from build123d import *

# Parameters (mm, degrees)
BODY_DEPTH                    = 6.35
HANDLE_DEPTH                  = 6.35
SKETCH11_R                    = 5
LOCKING_MECHANISM_HOLES_DEPTH = 6.36
FILLET1_R                     = 40
FILLET2_R                     = 40
SKETCH12_W                    = 10
SKETCH12_H                    = 30
BOSS_EXTRUDE1_DEPTH           = 4


with BuildPart() as part:
    # Sketch1 → Body (new body)
    with BuildSketch(Plane(origin=(0, 0, 0), x_dir=(1, 0, 0), z_dir=(0, 1, 0))):
        Polygon((0, 0), (294, 0), (336.996020767, 43.003978862), (336.996020767, 337.003978862), (217, 456.999999629), (77, 456.999999629), (-42.996020767, 337.003978862), (-42.996020767, 43.003978862), align=None)
    extrude(amount=BODY_DEPTH)

    # Sketch2 → Handle (cut)
    with BuildSketch(Plane(origin=(0, 6.35, 0), x_dir=(1, 0, 0), z_dir=(0, 1, 0))):
        with BuildLine():
            Line((112.35, 441.799999629), (181.65, 441.799999629))
            ThreePointArc((181.65, 441.799999629), (197.5, 425.949999629), (181.65, 410.099999629))
            Line((181.65, 410.099999629), (112.35, 410.099999629))
            ThreePointArc((112.35, 410.099999629), (96.5, 425.949999629), (112.35, 441.799999629))
        make_face()
    extrude(amount=-HANDLE_DEPTH, mode=Mode.SUBTRACT)

    # Sketch11 → Locking Mechanism Holes (cut)
    with BuildSketch(Plane(origin=(0, 6.35, 0), x_dir=(1, 0, 0), z_dir=(0, 1, 0))):
        with Locations(Location((221.65, 421.999999629, 0), (0, 0, 270))):
            Circle(SKETCH11_R)
        with Locations(Location((72.35, 421.999999629, 0), (0, 0, 270))):
            Circle(SKETCH11_R)
    extrude(amount=-LOCKING_MECHANISM_HOLES_DEPTH, mode=Mode.SUBTRACT)

    # Fillet1
    fillet1_edges = [part.edges().sort_by_distance(p)[0] for p in [
        (77, 3.175, -456.999999629),
        (217, 3.175, -456.999999629),
    ]]
    fillet(fillet1_edges, radius=FILLET1_R)

    # Fillet2
    fillet2_edges = [part.edges().sort_by_distance(p)[0] for p in [
        (-42.996020767, 3.175, -43.003978862),
        (-42.996020767, 3.175, -337.003978862),
        (336.996020767, 3.175, -337.003978862),
        (336.996020767, 3.175, -43.003978862),
        (294, 3.175, 0),
        (0, 3.175, 0),
    ]]
    fillet(fillet2_edges, radius=FILLET2_R)

    # Sketch12 → Boss-Extrude1 (add)
    with BuildSketch(Plane.XZ):
        with Locations((252.4, -251.999999629)):
            Rectangle(SKETCH12_W, SKETCH12_H)
        with Locations((41.6, -131.999999629)):
            Rectangle(SKETCH12_W, SKETCH12_H)
        with Locations((41.6, -251.999999629)):
            Rectangle(SKETCH12_W, SKETCH12_H)
        with Locations((252.4, -131.999999629)):
            Rectangle(SKETCH12_W, SKETCH12_H)
    extrude(amount=BOSS_EXTRUDE1_DEPTH)


solid = part.part
Here's how the part is built. I have some questions about the finished solid (model axes, mm). A direction names the side the tool comes from. Give positions to 0.01 mm unless a question says otherwise; leave off trailing zeros. Order: outer loops, then holes, each group sorted by start corner. A loop starts at its lowest first (then second) coordinate and runs counter-clockwise, first axis right, second up. Notation, with made-up numbers: (34.5, 57) -> (57.5, 57) arc R22 ccw to (57.5, 75) -> close; hole circle Ø9 at (69, 49). An arc over 180 degrees is marked (long way). Use a Markdown table: item, result. Add a question column.
Item 1: I need wall thicknesses on line 1 (X direction, y = 5, z = -422); line 2 (Y direction, x = 109, z = -276.5); line 3 (Z direction, x = 165.5, y = 4). Which ranges of each line are inside material? Lowest first, please.
Item 2: Imagine slicing it at D-D on z = -123. Please give me the cut outline in (x, y), plus the area to 3 significant figures.
Item 3: Imagine slicing it at A-A on x = 164.5. Please give me the cut outline in (y, z), plus the area to 3 significant figures.
Item 4: Will these pins go through, and if not, where does the flat tip stop? pin 1 (2 mm diameter, centred on x = 124.5, y = 0, fed in from +Z); pin 2 (1.2 mm diameter, centred on y = -1, z = -258.5, fed in from +X); pin 3 (1.2 mm diameter, centred on y = -2.5, z = -128, fed in from -X); pin 4 (1.2 mm diameter, centred on x = 39.5, y = -2, fed in from +Z).
Item 5: Imagine slicing it at C-C on z = -422. Please give me the cut outline in (x, y), plus the area to 4 significant figures.
Item 6: Imagine slicing it at B-B on y = -2. Please give me the cut outline in (x, z).
Item 7: For faces 4 (the face through (333.866, 3.219, -335.946)), 5 (the face through (96.504, 3.219, -425.601)), which set-ups out of +Z, -Z, +X, -X, +Y, -Y let a thin tool reach every point of the face, with its end or its side?
Item 8: If we mould it in two halves opening along X, with no side actions, what happens to faces 1 (the face through (-39.866, 3.219, -335.946)), 2 (the face through (197.496, 3.219, -426.299)), 3 (the face through (278, 3, -396))? For each: pulls with the +X half, pulls with the -X half, needs draft (parallel to the pull), parting line crosses it, or undercut.
Data:
| question | item | result |
|---|---|---|
| 1 | line 1 | x = 42 to 67.35, 77.35 to 97, 197 to 216.65, 226.65 to 252 |
| 1 | line 2 | y = 0 to 6.35 |
| 1 | line 3 | z = -457 to -441.8, -410.1 to 0 |
| 2 | outline | (-43, 0) -> (36.6, 0) -> (36.6, -4) -> (46.6, -4) -> (46.6, 0) -> (247.4, 0) -> (247.4, -4) -> (257.4, -4) -> (257.4, 0) -> (337, 0) -> (337, 6.35) -> (-43, 6.35) -> close |
| 2 | area | 2,490 mm² |
| 3 | outline | (0, -457) -> (6.35, -457) -> (6.35, -441.8) -> (0, -441.8) -> close; (0, -410.1) -> (6.35, -410.1) -> (6.35, 0) -> (0, 0) -> close |
| 3 | area | 2,700 mm² |
| 4 | pin 1 | stops at z = 0 |
| 4 | pin 2 | stops at x = 257.4 |
| 4 | pin 3 | stops at x = 36.6 |
| 4 | pin 4 | stops at z = -117 |
| 5 | outline | (42, 0) -> (67.35, 0) -> (67.35, 6.35) -> (42, 6.35) -> close; (77.35, 0) -> (97, 0) -> (97, 6.35) -> (77.35, 6.35) -> close; (197, 0) -> (216.65, 0) -> (216.65, 6.35) -> (197, 6.35) -> close; (226.65, 0) -> (252, 0) -> (252, 6.35) -> (226.65, 6.35) -> close |
| 5 | area | 571.5 mm² |
| 6 | outline | (36.6, -267) -> (46.6, -267) -> (46.6, -237) -> (36.6, -237) -> close; (36.6, -147) -> (46.6, -147) -> (46.6, -117) -> (36.6, -117) -> close; (247.4, -267) -> (257.4, -267) -> (257.4, -237) -> (247.4, -237) -> close; (247.4, -147) -> (257.4, -147) -> (257.4, -117) -> (247.4, -117) -> close |
| 7 | face 4 | -Z, +X, +Y, -Y |
| 7 | face 5 | +Y, -Y |
| 8 | face 1 | pulls with the -X half |
| 8 | face 2 | undercut |
| 8 | face 3 | pulls with the +X half |
